```python
from build123d import *

# Parameters (mm, degrees)
SKETCH_W      = 100
SKETCH_H      = 100
PAD_DEPTH     = 15
FILLET_R      = 10
FILLET001_R   = 10
FILLET002_R   = 10
FILLET003_R   = 10
SKETCH001_R   = 4.05
SKETCH001_R_2 = 3.05
SKETCH001_R_3 = 2.05
SKETCH001_R_4 = 1.6
POCKET_DEPTH  = 6


with BuildPart() as part:
    # Sketch → Pad (new body)
    with BuildSketch(Plane.XY):
        with Locations((50, 50)):
            Rectangle(SKETCH_W, SKETCH_H)
    extrude(amount=PAD_DEPTH)

    # Fillet
    fillet_edges = [part.edges().sort_by_distance(p)[0] for p in [
        (0, 0, 7.5),
    ]]
    fillet(fillet_edges, radius=FILLET_R)

    # Fillet001
    fillet001_edges = [part.edges().sort_by_distance(p)[0] for p in [
        (100, 0, 7.5),
    ]]
    fillet(fillet001_edges, radius=FILLET001_R)

    # Fillet002
    fillet002_edges = [part.edges().sort_by_distance(p)[0] for p in [
        (100, 100, 7.5),
    ]]
    fillet(fillet002_edges, radius=FILLET002_R)

    # Fillet003
    fillet003_edges = [part.edges().sort_by_distance(p)[0] for p in [
        (0, 100, 7.5),
    ]]
    fillet(fillet003_edges, radius=FILLET003_R)

    # Sketch001 (on Face6 of Pad) → Pocket (cut)
    with BuildSketch(Plane.XY.offset(15)):
        with Locations((15, 15)):
            Circle(SKETCH001_R)
        with Locations((15, 35)):
            Circle(SKETCH001_R)
        with Locations((15, 55)):
            Circle(SKETCH001_R)
        with Locations((15, 75)):
            Circle(SKETCH001_R)
        with Locations((35, 15)):
            Circle(SKETCH001_R_2)
        with Locations((35, 25)):
            Circle(SKETCH001_R_2)
        with Locations((35, 35)):
            Circle(SKETCH001_R_2)
        with Locations((35, 45)):
            Circle(SKETCH001_R_2)
        with Locations((35, 55)):
            Circle(SKETCH001_R_2)
        with Locations((35, 65)):
            Circle(SKETCH001_R_2)
        with Locations((35, 75)):
            Circle(SKETCH001_R_2)
        with Locations((35, 85)):
            Circle(SKETCH001_R_2)
        with Locations((50, 15)):
            Circle(SKETCH001_R_3)
        with Locations((50, 25)):
            Circle(SKETCH001_R_3)
        with Locations((50, 35)):
            Circle(SKETCH001_R_3)
        with Locations((50, 45)):
            Circle(SKETCH001_R_3)
        with Locations((50, 55)):
            Circle(SKETCH001_R_3)
        with Locations((50, 65)):
            Circle(SKETCH001_R_3)
        with Locations((50, 75)):
            Circle(SKETCH001_R_3)
        with Locations((50, 85)):
            Circle(SKETCH001_R_3)
        with Locations((65, 15)):
            Circle(SKETCH001_R_4)
        with Locations((65, 22)):
            Circle(SKETCH001_R_4)
        with Locations((65, 29)):
            Circle(SKETCH001_R_4)
        with Locations((65, 36)):
            Circle(SKETCH001_R_4)
        with Locations((65, 43)):
            Circle(SKETCH001_R_4)
        with Locations((65, 50)):
            Circle(SKETCH001_R_4)
        with Locations((65, 57)):
            Circle(SKETCH001_R_4)
        with Locations((65, 64)):
            Circle(SKETCH001_R_4)
        with Locations((65, 71)):
            Circle(SKETCH001_R_4)
        with Locations((65, 78)):
            Circle(SKETCH001_R_4)
        with Locations((65, 85)):
            Circle(SKETCH001_R_4)
        with Locations((80, 15)):
            Circle(SKETCH001_R_2)
        with Locations((80, 25)):
            Circle(SKETCH001_R_2)
        with Locations((80, 35)):
            Circle(SKETCH001_R_2)
        with Locations((80, 45)):
            Circle(SKETCH001_R_2)
        with Locations((80, 55)):
            Circle(SKETCH001_R_2)
        with Locations((80, 65)):
            Circle(SKETCH001_R_2)
        with Locations((80, 75)):
            Circle(SKETCH001_R_2)
        with Locations((80, 85)):
            Circle(SKETCH001_R_2)
    extrude(amount=-POCKET_DEPTH, mode=Mode.SUBTRACT)


solid = part.part
```
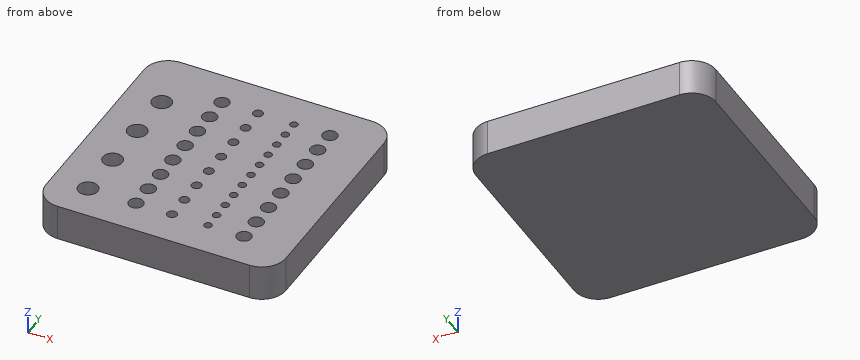
The model under review builds one solid part; all positions refer to its coordinate system, in mm. Coordinates: 2 decimals unless noted, no trailing zeros. Write each loop counter-clockwise with the first axis right and the second up, starting at its lowest first coordinate (ties: lowest second). Pieces come first, ordered by that corner, then holes.
1) We need section B-B on x = 15. State the section outline as (y, z) points.
2) We need section A-A on y = 15. State the section outline as (x, z) points.
3) To check wall thickness, follow probe 1 along Z at (x, y) = (33.5, 14.5); probe 2 along Y at (x, z) = (9, 2.25); probe 3 along X at (y, z) = (21, 12). State the ranges of each line that lie inside material, in increasing order.
4) Clearance check with a flat-ended pin moving along its axis: pin 1 Ø4 at (x, y) = (16, 55) entering from +Z. State where the tip first meets the part, or that it passes through.
5) We need section D-D on y = 25. State the section outline as (x, z) points, then the cut area to 3 significant figures.
6) We need section C-C on z = 11.25. Count the separate pieces of the cut face and the enclosed holes in it, then the cut area to 3 significant figures.
Answer list:
1. outline: (0, 0) - (100, 0) - (100, 15) - (79.05, 15) - (79.05, 9) - (70.95, 9) - (70.95, 15) - (59.05, 15) - (59.05, 9) - (50.95, 9) - (50.95, 15) - (39.05, 15) - (39.05, 9) - (30.95, 9) - (30.95, 15) - (19.05, 15) - (19.05, 9) - (10.95, 9) - (10.95, 15) - (0, 15) - close
2. outline: (0, 0) - (100, 0) - (100, 15) - (83.05, 15) - (83.05, 9) - (76.95, 9) - (76.95, 15) - (66.6, 15) - (66.6, 9) - (63.4, 9) - (63.4, 15) - (52.05, 15) - (52.05, 9) - (47.95, 9) - (47.95, 15) - (38.05, 15) - (38.05, 9) - (31.95, 9) - (31.95, 15) - (19.05, 15) - (19.05, 9) - (10.95, 9) - (10.95, 15) - (0, 15) - close
3. probe 1: z = 0 to 9
3. probe 2: y = 0.05 to 99.95
3. probe 3: x = 0 to 63.75, 66.25 to 100
4. pin 1: stops at z = 9
5. outline: (0, 0) - (100, 0) - (100, 15) - (83.05, 15) - (83.05, 9) - (76.95, 9) - (76.95, 15) - (52.05, 15) - (52.05, 9) - (47.95, 9) - (47.95, 15) - (38.05, 15) - (38.05, 9) - (31.95, 9) - (31.95, 15) - (0, 15) - close
5. area: 1,400 mm2
6. separate pieces: 1
6. enclosed holes: 39
6. area: 9,050 mm2
